from build123d import *

# Parameters (mm, degrees)
SKETCH2_W                   = 60
SKETCH2_H                   = 80
BOSS_EXTRUDE2_DEPTH         = 16
SKETCH6_W                   = 52
SKETCH6_H                   = 72
CUT_EXTRUDE1_DEPTH          = 12
CUT_EXTRUDE2_DEPTH          = 16
CUT_EXTRUDE2_DEPTH_BACK     = 106
SKETCH7_W                   = 22
SKETCH7_H                   = 8
SKETCH8_W                   = 4
SKETCH8_H                   = 10
BOSS_EXTRUDE3_DEPTH         = 12
FILLET1_RADIUS              = 5
FILLET1_LENGTH              = 4
FILLET2_RADIUS              = 5
FILLET2_LENGTH              = 4
FILLET3_RADIUS              = 5
FILLET3_LENGTH              = 4
FILLET4_RADIUS              = 5
FILLET4_LENGTH              = 4
BOSS_EXTRUDE4_START         = -2
SKETCH9_R                   = 2.5
BOSS_EXTRUDE4_DEPTH         = 26
MIRROR2_START               = -2
MIRROR2_COPY_1_SKETCH_R     = 2.5
MIRROR2_COPY_1_DEPTH        = 26
FILLET1_OF_MIRROR2_2_RADIUS = 5
FILLET1_OF_MIRROR2_2_LENGTH = 4
FILLET2_OF_MIRROR2_2_RADIUS = 5
FILLET2_OF_MIRROR2_2_LENGTH = 4
FILLET3_OF_MIRROR2_2_RADIUS = 5
FILLET3_OF_MIRROR2_2_LENGTH = 4
FILLET4_OF_MIRROR2_2_RADIUS = 5
FILLET4_OF_MIRROR2_2_LENGTH = 4
SKETCH10_W                  = 20
SKETCH10_H                  = 1
BOSS_EXTRUDE5_DEPTH         = 2.999340988
SKETCH12_W                  = 20
SKETCH12_H                  = 3
BOSS_EXTRUDE6_DEPTH         = 3
FILLET6_RADIUS              = 1.5
FILLET6_LENGTH              = 20
FILLET7_R                   = 2
FILLET8_R                   = 2
FILLET9_R                   = 2
FILLET10_R                  = 2
FILLET11_R                  = 2


with BuildPart() as part:
    # Sketch2 → Boss-Extrude2 (new body)
    with BuildSketch(Plane(origin=(0, 0, 0), x_dir=(1, 0, 0), z_dir=(0, 1, 0))):
        Rectangle(SKETCH2_W, SKETCH2_H)
    extrude(amount=BOSS_EXTRUDE2_DEPTH)

    # Sketch6 → Cut-Extrude1 (cut)
    with BuildSketch(Plane(origin=(0, 16, 0), x_dir=(1, 0, 0), z_dir=(0, 1, 0))):
        Rectangle(SKETCH6_W, SKETCH6_H)
    extrude(amount=-CUT_EXTRUDE1_DEPTH, mode=Mode.SUBTRACT)

    # Sketch7 → Cut-Extrude2 (cut, two sides: drawn at the far end of the back side and taken through both)
    with BuildSketch(Plane(origin=(0, 0, -40), x_dir=(-1, 0, 0), z_dir=(0, 0, -1)).offset(-CUT_EXTRUDE2_DEPTH_BACK)):
        with Locations((-14, 8)):
            Rectangle(SKETCH7_W, SKETCH7_H)
        with Locations((14, 8)):
            Rectangle(SKETCH7_W, SKETCH7_H)
    extrude(amount=CUT_EXTRUDE2_DEPTH + CUT_EXTRUDE2_DEPTH_BACK, mode=Mode.SUBTRACT)

    # Sketch8 → Boss-Extrude3 (add)
    with BuildSketch(Plane(origin=(30, 0, 0), x_dir=(0, 0, -1), z_dir=(1, 0, 0))):
        with Locations((-33, 8.303078398)):
            Rectangle(SKETCH8_W, SKETCH8_H)
        with Locations((-7, 8.355173675)):
            Rectangle(SKETCH8_W, SKETCH8_H)
        with Locations((7, 8.355173675)):
            Rectangle(SKETCH8_W, SKETCH8_H)
        with Locations((33, 8.303078398)):
            Rectangle(SKETCH8_W, SKETCH8_H)
    boss_extrude3 = extrude(amount=BOSS_EXTRUDE3_DEPTH)

    # Fillet1: full round fillet: the end face becomes a half cylinder, R = half its width
    fillet1_face = Plane((42, 8.303078398, 33), x_dir=(0, 0, 1), z_dir=(1, 0, 0))  # on the end face: x along it, z out of the body
    fillet1_slab = fillet1_face.offset(-FILLET1_RADIUS / 2) * Box(FILLET1_LENGTH, 2 * FILLET1_RADIUS, FILLET1_RADIUS, mode=Mode.PRIVATE)  # the body's end, R deep
    fillet1_round = Plane((37, 8.303078398, 33), x_dir=(1, 0, 0), z_dir=(0, 0, 1)) * Cylinder(FILLET1_RADIUS, FILLET1_LENGTH, mode=Mode.PRIVATE)  # its axis R under the face
    add(fillet1_slab - fillet1_round, mode=Mode.SUBTRACT)

    # Fillet2: full round fillet: the end face becomes a half cylinder, R = half its width
    fillet2_face = Plane((42, 8.355173675, 7), x_dir=(0, 0, 1), z_dir=(1, 0, 0))  # on the end face: x along it, z out of the body
    fillet2_slab = fillet2_face.offset(-FILLET2_RADIUS / 2) * Box(FILLET2_LENGTH, 2 * FILLET2_RADIUS, FILLET2_RADIUS, mode=Mode.PRIVATE)  # the body's end, R deep
    fillet2_round = Plane((37, 8.355173675, 7), x_dir=(1, 0, 0), z_dir=(0, 0, 1)) * Cylinder(FILLET2_RADIUS, FILLET2_LENGTH, mode=Mode.PRIVATE)  # its axis R under the face
    add(fillet2_slab - fillet2_round, mode=Mode.SUBTRACT)

    # Fillet3: full round fillet: the end face becomes a half cylinder, R = half its width
    fillet3_face = Plane((42, 8.355173675, -7), x_dir=(0, 0, -1), z_dir=(1, 0, 0))  # on the end face: x along it, z out of the body
    fillet3_slab = fillet3_face.offset(-FILLET3_RADIUS / 2) * Box(FILLET3_LENGTH, 2 * FILLET3_RADIUS, FILLET3_RADIUS, mode=Mode.PRIVATE)  # the body's end, R deep
    fillet3_round = Plane((37, 8.355173675, -7), x_dir=(1, 0, 0), z_dir=(0, 0, -1)) * Cylinder(FILLET3_RADIUS, FILLET3_LENGTH, mode=Mode.PRIVATE)  # its axis R under the face
    add(fillet3_slab - fillet3_round, mode=Mode.SUBTRACT)

    # Fillet4: full round fillet: the end face becomes a half cylinder, R = half its width
    fillet4_face = Plane((42, 8.303078398, -33), x_dir=(0, 0, -1), z_dir=(1, 0, 0))  # on the end face: x along it, z out of the body
    fillet4_slab = fillet4_face.offset(-FILLET4_RADIUS / 2) * Box(FILLET4_LENGTH, 2 * FILLET4_RADIUS, FILLET4_RADIUS, mode=Mode.PRIVATE)  # the body's end, R deep
    fillet4_round = Plane((37, 8.303078398, -33), x_dir=(1, 0, 0), z_dir=(0, 0, -1)) * Cylinder(FILLET4_RADIUS, FILLET4_LENGTH, mode=Mode.PRIVATE)  # its axis R under the face
    add(fillet4_slab - fillet4_round, mode=Mode.SUBTRACT)

    # Sketch9 → Boss-Extrude4 (add)
    with BuildSketch(Plane(origin=(0, 0, 31), x_dir=(-1, 0, 0), z_dir=(0, 0, -1)).offset(BOSS_EXTRUDE4_START)):
        with Locations(Location((-37, 8.303078398, 0), (0, 0, 180))):
            Circle(SKETCH9_R)
    boss_extrude4 = extrude(amount=BOSS_EXTRUDE4_DEPTH)

    # Mirror1: Boss-Extrude4 across plane
    add(boss_extrude4.mirror(Plane(origin=(0, 0, 0), x_dir=(1, 0, 0), z_dir=(0, 0, -1))))

    # Mirror2: Boss-Extrude3, Boss-Extrude4 across plane
    add(boss_extrude3.mirror(Plane(origin=(0, 0, 0), x_dir=(0, 0, 1), z_dir=(1, 0, 0))))
    add(boss_extrude4.mirror(Plane(origin=(0, 0, 0), x_dir=(0, 0, 1), z_dir=(1, 0, 0))))

    # Mirror2 copy 1 sketch → Mirror2 copy 1 (add)
    with BuildSketch(Plane.XY.offset(-31).offset(MIRROR2_START)):
        with Locations(Location((-37, 8.303078398, 0), (0, 0, 180))):
            Circle(MIRROR2_COPY_1_SKETCH_R)
    extrude(amount=MIRROR2_COPY_1_DEPTH)

    # Fillet1 of Mirror2 2: full round fillet: the end face becomes a half cylinder, R = half its width
    fillet1_of_mirror2_2_face = Plane((-42, 8.303078398, 33), x_dir=(0, 0, 1), z_dir=(-1, 0, 0))  # on the end face: x along it, z out of the body
    fillet1_of_mirror2_2_slab = fillet1_of_mirror2_2_face.offset(-FILLET1_OF_MIRROR2_2_RADIUS / 2) * Box(FILLET1_OF_MIRROR2_2_LENGTH, 2 * FILLET1_OF_MIRROR2_2_RADIUS, FILLET1_OF_MIRROR2_2_RADIUS, mode=Mode.PRIVATE)  # the body's end, R deep
    fillet1_of_mirror2_2_round = Plane((-37, 8.303078398, 33), x_dir=(-1, 0, 0), z_dir=(0, 0, 1)) * Cylinder(FILLET1_OF_MIRROR2_2_RADIUS, FILLET1_OF_MIRROR2_2_LENGTH, mode=Mode.PRIVATE)  # its axis R under the face
    add(fillet1_of_mirror2_2_slab - fillet1_of_mirror2_2_round, mode=Mode.SUBTRACT)

    # Fillet2 of Mirror2 2: full round fillet: the end face becomes a half cylinder, R = half its width
    fillet2_of_mirror2_2_face = Plane((-42, 8.355173675, 7), x_dir=(0, 0, 1), z_dir=(-1, 0, 0))  # on the end face: x along it, z out of the body
    fillet2_of_mirror2_2_slab = fillet2_of_mirror2_2_face.offset(-FILLET2_OF_MIRROR2_2_RADIUS / 2) * Box(FILLET2_OF_MIRROR2_2_LENGTH, 2 * FILLET2_OF_MIRROR2_2_RADIUS, FILLET2_OF_MIRROR2_2_RADIUS, mode=Mode.PRIVATE)  # the body's end, R deep
    fillet2_of_mirror2_2_round = Plane((-37, 8.355173675, 7), x_dir=(-1, 0, 0), z_dir=(0, 0, 1)) * Cylinder(FILLET2_OF_MIRROR2_2_RADIUS, FILLET2_OF_MIRROR2_2_LENGTH, mode=Mode.PRIVATE)  # its axis R under the face
    add(fillet2_of_mirror2_2_slab - fillet2_of_mirror2_2_round, mode=Mode.SUBTRACT)

    # Fillet3 of Mirror2 2: full round fillet: the end face becomes a half cylinder, R = half its width
    fillet3_of_mirror2_2_face = Plane((-42, 8.355173675, -7), x_dir=(0, 0, -1), z_dir=(-1, 0, 0))  # on the end face: x along it, z out of the body
    fillet3_of_mirror2_2_slab = fillet3_of_mirror2_2_face.offset(-FILLET3_OF_MIRROR2_2_RADIUS / 2) * Box(FILLET3_OF_MIRROR2_2_LENGTH, 2 * FILLET3_OF_MIRROR2_2_RADIUS, FILLET3_OF_MIRROR2_2_RADIUS, mode=Mode.PRIVATE)  # the body's end, R deep
    fillet3_of_mirror2_2_round = Plane((-37, 8.355173675, -7), x_dir=(-1, 0, 0), z_dir=(0, 0, -1)) * Cylinder(FILLET3_OF_MIRROR2_2_RADIUS, FILLET3_OF_MIRROR2_2_LENGTH, mode=Mode.PRIVATE)  # its axis R under the face
    add(fillet3_of_mirror2_2_slab - fillet3_of_mirror2_2_round, mode=Mode.SUBTRACT)

    # Fillet4 of Mirror2 2: full round fillet: the end face becomes a half cylinder, R = half its width
    fillet4_of_mirror2_2_face = Plane((-42, 8.303078398, -33), x_dir=(0, 0, -1), z_dir=(-1, 0, 0))  # on the end face: x along it, z out of the body
    fillet4_of_mirror2_2_slab = fillet4_of_mirror2_2_face.offset(-FILLET4_OF_MIRROR2_2_RADIUS / 2) * Box(FILLET4_OF_MIRROR2_2_LENGTH, 2 * FILLET4_OF_MIRROR2_2_RADIUS, FILLET4_OF_MIRROR2_2_RADIUS, mode=Mode.PRIVATE)  # the body's end, R deep
    fillet4_of_mirror2_2_round = Plane((-37, 8.303078398, -33), x_dir=(-1, 0, 0), z_dir=(0, 0, -1)) * Cylinder(FILLET4_OF_MIRROR2_2_RADIUS, FILLET4_OF_MIRROR2_2_LENGTH, mode=Mode.PRIVATE)  # its axis R under the face
    add(fillet4_of_mirror2_2_slab - fillet4_of_mirror2_2_round, mode=Mode.SUBTRACT)

    # Sketch10 → Boss-Extrude5 (add)
    with BuildSketch(Plane(origin=(-26, 0, 0), x_dir=(0, 0, -1), z_dir=(1, 0, 0))):
        with Locations((0, 12.5)):
            Rectangle(SKETCH10_W, SKETCH10_H)
    extrude(amount=BOSS_EXTRUDE5_DEPTH)

    # Sketch12 → Boss-Extrude6 (add)
    with BuildSketch(Plane.ZY.offset(-26)):
        with Locations((0, 14.5)):
            Rectangle(SKETCH12_W, SKETCH12_H)
    extrude(amount=BOSS_EXTRUDE6_DEPTH)

    # Sketch13 → Revolve1 (revolve)
    with BuildSketch(Plane.XY.offset(10)):
        with BuildLine():
            Line((23.50027011, 14.5), (25.49972989, 14.5))
            ThreePointArc((25.49972989, 14.5), (24.5, 13.50027011), (23.50027011, 14.5))
        make_face()
    revolve1 = revolve(axis=Axis((23.50027011, 14.5, 10), (1, 0, 0)))

    # Mirror3: Revolve1 across plane
    add(revolve1.mirror(Plane(origin=(0, 0, 0), x_dir=(1, 0, 0), z_dir=(0, 0, -1))))

    # Fillet6: full round fillet: the end face becomes a half cylinder, R = half its width
    fillet6_face = Plane((23, 14.5, 0), x_dir=(0, 0, -1), z_dir=(-1, 0, 0))  # on the end face: x along it, z out of the body
    fillet6_slab = fillet6_face.offset(-FILLET6_RADIUS / 2) * Box(FILLET6_LENGTH, 2 * FILLET6_RADIUS, FILLET6_RADIUS, mode=Mode.PRIVATE)  # the body's end, R deep
    fillet6_round = Plane((24.5, 14.5, 0), x_dir=(-1, 0, 0), z_dir=(0, 0, -1)) * Cylinder(FILLET6_RADIUS, FILLET6_LENGTH, mode=Mode.PRIVATE)  # its axis R under the face
    add(fillet6_slab - fillet6_round, mode=Mode.SUBTRACT)

    # Fillet7
    fillet7_edges = [part.edges().sort_by_distance(p)[0] for p in [
        (-30, 16, 0),
    ]]
    fillet(fillet7_edges, radius=FILLET7_R)

    # Fillet8
    fillet8_edges = [part.edges().sort_by_distance(p)[0] for p in [
        (1, 16, -40),
        (-30, 7, -40),
        (-29.414213562, 15.414213562, -40),
    ]]
    fillet(fillet8_edges, radius=FILLET8_R)

    # Fillet9
    fillet9_edges = [part.edges().sort_by_distance(p)[0] for p in [
        (30, 16, 1),
        (30, 7, -40),
        (30, 15.414213562, -39.414213562),
    ]]
    fillet(fillet9_edges, radius=FILLET9_R)

    # Fillet10
    fillet10_edges = [part.edges().sort_by_distance(p)[0] for p in [
        (0, 16, 40),
        (-30, 7, 40),
        (-29.414213562, 15.414213562, 40),
        (30, 7, 40),
        (29.414213562, 15.414213562, 40),
    ]]
    fillet(fillet10_edges, radius=FILLET10_R)

    # Fillet11
    fillet11_edges = [part.edges().sort_by_distance(p)[0] for p in [
        (0, 0, -40),
        (-30, 0, 0),
        (-29.414213562, 0, -39.414213562),
        (30, 0, 0),
        (29.414213562, 0, -39.414213562),
        (0, 0, 40),
        (29.414213562, 0, 39.414213562),
        (-29.414213562, 0, 39.414213562),
    ]]
    fillet(fillet11_edges, radius=FILLET11_R)


solid = part.part
CAD build for the part. Positions are in the model's coordinates, mm. A direction names the side the tool comes from. Coordinates: 2 decimals unless noted, no trailing zeros. Write each loop counter-clockwise with the first axis right and the second up, starting at its lowest first coordinate (ties: lowest second). Pieces come first, ordered by that corner, then holes. Notation, with made-up numbers: M 66.25,30 L 72.25,30 A33 ccw 72.25,58 Z; hole C -7,-32 d6. An arc over 180 degrees is marked long. Answer as a JSON object with one key per item and string values. Group by question number.
1) Pin check, flat tips, straight feed: pin 1 Ø5 at (x, y) = (34, 10) entering from -Z; pin 2 Ø3 at (x, y) = (-30, 7) entering from -Z; pin 3 Ø4 at (x, z) = (17, 22.5) entering from +Y. Stop position of each tip, or through.
2) Saw through at B-B (z = 34). Write the cut outline in (x, y).
3) Tool access for faces 5 (the face through (33, 3.303, 33)), 6 (the face through (3, 8, -38)): list every direction of +Z, -Z, +X, -X, +Y, -Y with a clear straight run to the whole face (end or side of a thin tool).
4) Saw through at A-A (x = -15). Write the cut outline in (y, z).
5) Saw through at D-D (z = 12.5). Write the cut outline in (x, y).
6) Mould opens along Y. For faces 1 (the face through (-25, 12, 0)), 2 (the face through (23, 14.5, -0.1)), 3 (the face through (-39.4, 7.6, -20.2)), 4 (the face through (-33, 3.303, 33)) say: +Y half, -Y half, draft (parallel to the pull), parting line (faces both ways), or undercut.
7) Wall check: line 1 (X direction, y = 11.25, z = 36.5); line 2 (Z direction, x = -34, y = 10.5); line 3 (X direction, y = 4.25, z = -4.5). Give the ranges that are in metal, low to high. Write a range as from..to.
8) Saw through at C-C (y = 9.75). Give the number of separate pieces and of enclosed holes in the cut face, plus the area to 3 significant figures.
Values follow:
{
 "1": {"pin 1": "stops at z = -35", "pin 2": "stops at z = -39.94", "pin 3": "stops at y = 4"},
 "2": {"outline": "M -37,3.3 L -30,3.3 L -30,2 A2 ccw -28,0 L 28,0 A2 ccw 30,2 L 30,3.3 L 37,3.3 A5 ccw 37,13.3 L 30,13.3 L 30,14 A2 ccw 28,16 L 26,16 L 26,4 L -26,4 L -26,16 L -28,16 A2 ccw -30,14 L -30,13.3 L -37,13.3 A5 ccw Z"},
 "3": {"face 5": "+Z, -Z, +X, -Y", "face 6": "+Z, -Z"},
 "4": {"outline": "M 0,-38 A2 ccw 2,-40 L 4,-40 L 4,40 L 2,40 A2 ccw 0,38 Z; M 12,-40 L 14,-40 A2 ccw 16,-38 L 16,-36 L 12,-36 Z; M 12,36 L 16,36 L 16,38 A2 ccw 14,40 L 12,40 Z"},
 "5": {"outline": "C -37,8.3 d5; M -30,2 A2 ccw -28,0 L 28,0 A2 ccw 30,2 L 30,14 A2 ccw 28,16 L 26,16 L 26,4 L -26,4 L -26,16 L -28,16 A2 ccw -30,14 Z; C 37,8.3 d5"},
 "6": {"face 1": "undercut", "face 2": "undercut", "face 3": "parting line", "face 4": "-Y half"},
 "7": {"line 1": "x = -30..-25, -3..3, 25..30", "line 2": "z = -35..-31, -9..-5, 5..9, 31..35", "line 3": "x = -30..-26, 26..30"},
 "8": {"separate pieces": "4", "enclosed holes": "4", "area": "1,440 mm2"}
}
